Geometry: final body of the model. Coordinates: model frame, mm. A direction names the side the tool comes from. Round coordinates to 2 decimals unless told otherwise and drop trailing zeros. Write each loop counter-clockwise with the first axis right and the second up, starting at its lowest first coordinate (ties: lowest second). Pieces come first, ordered by that corner, then holes. Notation, with made-up numbers: M -12,-25 L 3,-25 A20 cw 3,-19 Z; hole C 26,17.25 d7. An arc over 180 degrees is marked long. Put each result on its own line as item: value. Start each with the question number.
```python
from build123d import *

# Parameters (mm, degrees)
SKETCH1_W           = 166.5
SKETCH1_H           = 30.5
BOSS_EXTRUDE1_DEPTH = 24
SKETCH2_W           = 30
SKETCH2_H           = 10
CUT_EXTRUDE1_DEPTH  = 123.108559222
CUT_EXTRUDE2_DEPTH  = 118.768839527
FILLET1_R           = 2
FILLET2_R           = 13
SKETCH5_W           = 132.5
SKETCH5_H           = 22.5
CUT_EXTRUDE3_DEPTH  = 19
SKETCH6_R           = 7.5
CUT_EXTRUDE4_DEPTH  = 4
SKETCH7_W           = 13
SKETCH7_H           = 8.8
BOSS_EXTRUDE2_DEPTH = 22.5
SKETCH8_R           = 2
CUT_EXTRUDE5_DEPTH  = 13


with BuildPart() as part:
    # Sketch1 → Boss-Extrude1 (new body)
    with BuildSketch(Plane(origin=(0, 0, 0), x_dir=(1, 0, 0), z_dir=(0, 1, 0))):
        with Locations((-27.940150479, -29.14876881)):
            Rectangle(SKETCH1_W, SKETCH1_H)
    extrude(amount=BOSS_EXTRUDE1_DEPTH)

    # Sketch2 → Cut-Extrude1 (cut, through all)
    with BuildSketch(Plane.XZ):
        with Locations((40.309849521, 29.14876881)):
            Rectangle(SKETCH2_W, SKETCH2_H)
    extrude(amount=-CUT_EXTRUDE1_DEPTH, mode=Mode.SUBTRACT)

    # Sketch4 → Cut-Extrude2 (cut, through all)
    with BuildSketch(Plane(origin=(0, 0, 13.89876881), x_dir=(-1, 0, 0), z_dir=(0, 0, -1))):
        with BuildLine():
            Line((-26.315186332, 3.097371167), (-26.315186332, 0))
            Line((-26.315186332, 0), (-55.309849521, 0))
            Line((-55.309849521, 0), (-55.309849521, 12))
            Line((-55.309849521, 12), (-42.521374472, 12))
            ThreePointArc((-42.521374472, 12), (-31.784812397, 12.342604184), (-26.315186332, 3.097371167))
        make_face()
    extrude(amount=-CUT_EXTRUDE2_DEPTH, mode=Mode.SUBTRACT)

    # Fillet1
    fillet1_edges = [part.edges().sort_by_distance(p)[0] for p in [
        (55.309849521, 18, 44.39876881),
        (55.309849521, 18, 13.89876881),
    ]]
    fillet(fillet1_edges, radius=FILLET1_R)

    # Fillet2
    fillet2_edges = [part.edges().sort_by_distance(p)[0] for p in [
        (-42.437482073, 0, 44.39876881),
        (-42.437482073, 0, 13.89876881),
    ]]
    fillet(fillet2_edges, radius=FILLET2_R)

    # Sketch5 → Cut-Extrude3 (cut)
    with BuildSketch(Plane(origin=(0, 24, 0), x_dir=(1, 0, 0), z_dir=(0, 1, 0))):
        with Locations((-40.940150479, -29.14876881)):
            Rectangle(SKETCH5_W, SKETCH5_H)
    extrude(amount=-CUT_EXTRUDE3_DEPTH, mode=Mode.SUBTRACT)

    # Sketch6 → Cut-Extrude4 (cut)
    with BuildSketch(Plane.ZY.offset(111.190150479)):
        with Locations((29.14876881, 13.8)):
            Circle(SKETCH6_R)
    extrude(amount=-CUT_EXTRUDE4_DEPTH, mode=Mode.SUBTRACT)

    # Sketch7 → Boss-Extrude2 (add)
    with BuildSketch(Plane(origin=(0, 0, 40.39876881), x_dir=(-1, 0, 0), z_dir=(0, 0, -1))):
        with Locations((-12.376968122, 14.857402626)):
            Rectangle(SKETCH7_W, SKETCH7_H)
    extrude(amount=BOSS_EXTRUDE2_DEPTH)

    # Sketch8 → Cut-Extrude5 (cut)
    with BuildSketch(Plane(origin=(18.876968122, 0, 0), x_dir=(0, 0, -1), z_dir=(1, 0, 0))):
        with Locations((-29.14876881, 13.8)):
            Circle(SKETCH8_R)
    extrude(amount=-CUT_EXTRUDE5_DEPTH, mode=Mode.SUBTRACT)


solid = part.part
```
1) Ray query, probe 1 along X at (y, z) = (23, 19); probe 2 along X at (y, z) = (7.25, 21); probe 3 along X at (y, z) = (5.75, 29.5). Return the intervals inside material, ascending.
2) Access query for faces 1 (the face through (5.877, 17, 29)), 2 (the face through (40, 17, 34.149)), 3 (the face through (12, 10.457, 29)), 4 (the face through (26.315, 2, 36)). Directions: +Z, -Z, +X, -X, +Y, -Y. A direction counts if a zero-diameter tool reaches every point of the face in a straight line with its end or side. Return the directions, or none.
3) Draft query along Y for faces 5 (the face through (-44, 0, 29)), 6 (the face through (-109.22, 10.93, 36.08)), 7 (the face through (12.468, 13.034, 27.301)), 8 (the face through (55.31, 18, 20)). Return one class per face: +Y half, -Y half, draft (parallel to the pull), parting line (faces both ways), or undercut.
4) Section A-A, the plane x = -93.5. Output: boundary loops of the cut face in (y, z).
5) First-contact query: pin 1 (3 mm diameter, centred on x = 48.5, z = 37, fed in from -Y); pin 2 (5 mm diameter, centred on y = 6.5, z = 34.5, fed in from +X); pin 3 (6 mm diameter, centred on x = -64, y = 6.5, fed in from +Z). Flat tips, straight axial feed; report the tip coordinate or a pass-through.
Solved:
1. probe 1: x = -111.19 to -107.19, 25.31 to 55.31
1. probe 2: x = -111.19 to -107.19, 25.31 to 27.17
1. probe 3: x = -111.19 to -107.19
2. face 1: +Y
2. face 2: +X, +Y, -Y
2. face 3: none
2. face 4: +Z, -Z, +X, -Y
3. face 5: -Y half
3. face 6: undercut
3. face 7: undercut
3. face 8: draft
4. outline: M 0,26.9 A13 ccw 13,13.9 L 24,13.9 L 24,17.9 L 5,17.9 L 5,40.4 L 24,40.4 L 24,44.4 L 13,44.4 A13 ccw 0,31.4 Z
5. pin 1: stops at y = 12
5. pin 2: stops at x = 28.12
5. pin 3: stops at z = 43.92
